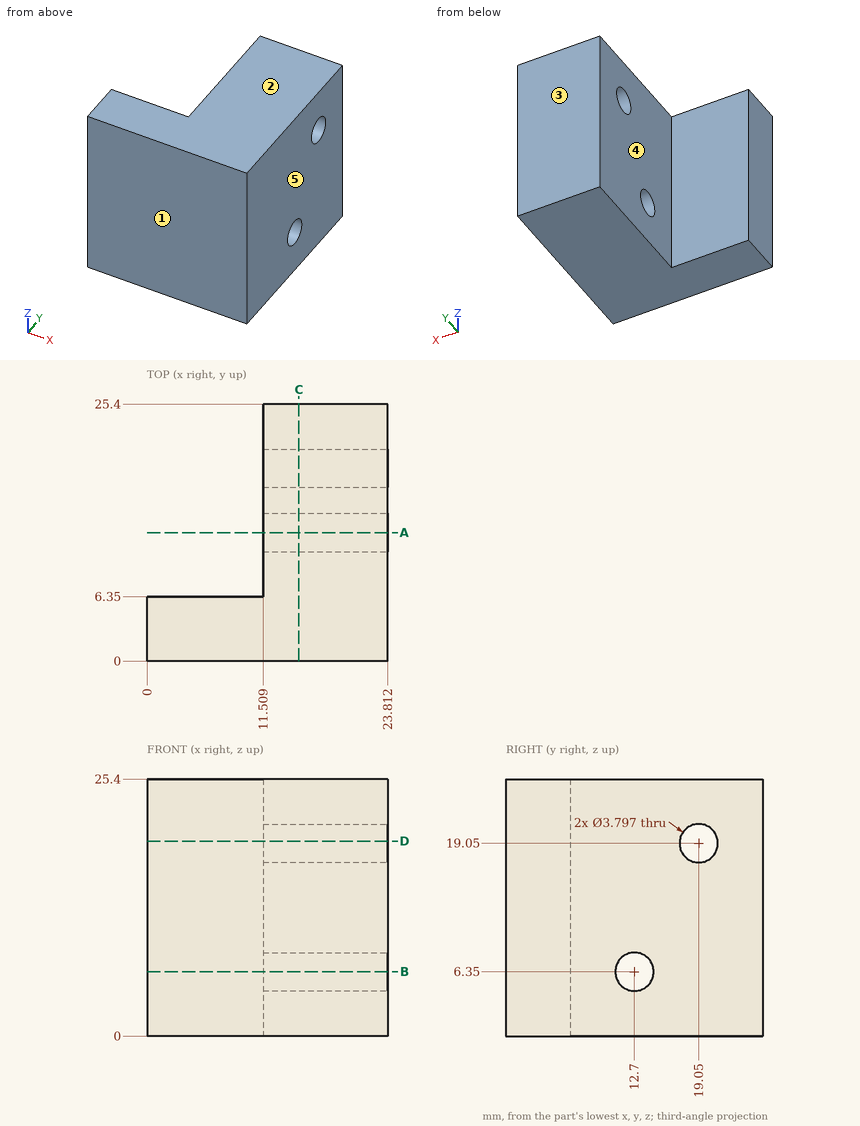
Source: three-view drawing plus pictorial views. Frame: mm from the lowest corner of the part. A direction names the side the tool comes from. Round coordinates to 2 decimals unless told otherwise and drop trailing zeros. Order: outer loops, then holes, each group sorted by start corner. A loop starts at its lowest first (then second) coordinate and runs counter-clockwise, first axis right, second up. Notation, with made-up numbers: (19.5, -26) -> (68.5, -26) arc R33 ccw to (68.5, 9) -> close; hole circle Ø8 at (59, -24). An arc over 180 degrees is marked (long way). Use CSV: the item, a comma, the result in double quotes. Start each with the question number.
1) Section B-B (z = 6.35). Return the cut outline in (x, y), and give its area (3 significant figures).
2) Draft query along Y for the marked faces 1, 2 and 3. Return one class per face: +Y half, -Y half, draft (parallel to the pull), parting line (faces both ways), or undercut.
3) Material intervals for line 1 along Y through (x, z) = (16, 6.35); line 2 along Y through (x, z) = (21, 19.05); line 3 along Z through (x, y) = (16.5, 12.7), sorted ascending. Write a range as from..to.
4) Section D-D (z = 19.25). Return the cut outline in (x, y).
5) First-contact query: pin 1 Ø6 at (y, z) = (12.7, 6.35) entering from -X; pin 2 Ø4 at (x, z) = (7.5, 12.5) entering from -Y; pin 3 Ø6 at (x, z) = (3, 19) entering from +Y. Flat tips, straight axial feed; report the tip coordinate or a pass-through.
6) Set-up query: the marked faces 4 and 5. Return all of +Z, -Z, +X, -X, +Y, -Y with unobstructed straight access to the full face (end or side cutting, diameter ignored); none if empty.
7) Section C-C (x = 15). Return the cut outline in (y, z).
8) Section A-A (y = 12.7). Return the cut outline in (x, z).
Returned:
1,outline,"(0, 0) -> (23.81, 0) -> (23.81, 10.8) -> (11.51, 10.8) -> (11.51, 6.35) -> (0, 6.35) -> close; (11.51, 14.6) -> (23.81, 14.6) -> (23.81, 25.4) -> (11.51, 25.4) -> close"
1,area,"339 mm²"
2,face 1,"-Y half"
2,face 2,"draft"
2,face 3,"+Y half"
3,line 1,"y = 0..10.8, 14.6..25.4"
3,line 2,"y = 0..17.15, 20.95..25.4"
3,line 3,"z = 0..4.45, 8.25..25.4"
4,outline,"(0, 0) -> (23.81, 0) -> (23.81, 17.16) -> (11.51, 17.16) -> (11.51, 6.35) -> (0, 6.35) -> close; (11.51, 20.94) -> (23.81, 20.94) -> (23.81, 25.4) -> (11.51, 25.4) -> close"
5,pin 1,"stops at x = 11.51"
5,pin 2,"stops at y = 0"
5,pin 3,"stops at y = 6.35"
6,face 4,"+Z, -Z, -X, +Y"
6,face 5,"+Z, -Z, +X, +Y, -Y"
7,outline,"(0, 0) -> (25.4, 0) -> (25.4, 25.4) -> (0, 25.4) -> close; hole circle Ø3.8 at (12.7, 6.35); hole circle Ø3.8 at (19.05, 19.05)"
8,outline,"(11.51, 0) -> (23.81, 0) -> (23.81, 4.45) -> (11.51, 4.45) -> close; (11.51, 8.25) -> (23.81, 8.25) -> (23.81, 25.4) -> (11.51, 25.4) -> close"
